from build123d import *

# Parameters (mm, degrees)
F0_W     = 20.5
F0_H     = 15.25
F0_W_2   = 18
F0_H_2   = 13
F0_R     = 3.125
F1_DEPTH = 2
F2_DEPTH = 5


# Not quite as in the source:
# - a fillet or chamfer that OpenCascade refuses, or shapes differently, is made with other operations: its cross-section is extruded or revolved along the edge and cut away or added


with BuildPart() as f1:
    # F0 (on Top) → F1 (new body)
    with BuildSketch(Plane.XY):
        Rectangle(F0_W, F0_H)
        Rectangle(F0_W_2, F0_H_2, mode=Mode.SUBTRACT)
        Rectangle(F0_W_2, F0_H_2)
        with Locations((-1.775, -3.075)):
            Circle(F0_R, mode=Mode.SUBTRACT)
        with Locations((5.475, -3.075)):
            Circle(F0_R, mode=Mode.SUBTRACT)
        with Locations((-5.475, 3.075)):
            Circle(F0_R, mode=Mode.SUBTRACT)
        with Locations((1.775, 3.075)):
            Circle(F0_R, mode=Mode.SUBTRACT)
    extrude(amount=F1_DEPTH)

    # F0 (on Top) → F2 (join)
    with BuildSketch(Plane.XY):
        Rectangle(F0_W_2, F0_H_2)
        with Locations((-1.775, -3.075)):
            Circle(F0_R, mode=Mode.SUBTRACT)
        with Locations((5.475, -3.075)):
            Circle(F0_R, mode=Mode.SUBTRACT)
        with Locations((-5.475, 3.075)):
            Circle(F0_R, mode=Mode.SUBTRACT)
        with Locations((1.775, 3.075)):
            Circle(F0_R, mode=Mode.SUBTRACT)
    extrude(amount=F2_DEPTH)

    # F3: fillet of radius 1 on 4 edges, made by hand

    # F3_s1 → F3_t2 (revolve, cut)
    with BuildSketch(Plane.XZ.offset(-3.075)):
        with BuildLine():
            ThreePointArc((-1.35, 5), (-2.0571067812, 4.7071067812), (-2.35, 4))
            Line((-2.35, 4), (-2.35, 5))
            Line((-2.35, 5), (-1.35, 5))
        make_face()
    revolve(axis=Axis((-5.475, 3.075, 5), (0, 0, 1)), mode=Mode.SUBTRACT)

    # F3_s3 → F3_t4 (revolve, cut)
    with BuildSketch(Plane.XZ.offset(-3.075)):
        with BuildLine():
            ThreePointArc((5.9, 5), (5.1928932188, 4.7071067812), (4.9, 4))
            Line((4.9, 4), (4.9, 5))
            Line((4.9, 5), (5.9, 5))
        make_face()
    revolve(axis=Axis((1.775, 3.075, 5), (0, 0, 1)), mode=Mode.SUBTRACT)

    # F3_s5 → F3_t6 (revolve, cut)
    with BuildSketch(Plane.XZ.offset(3.075)):
        with BuildLine():
            ThreePointArc((2.35, 5), (1.6428932188, 4.7071067812), (1.35, 4))
            Line((1.35, 4), (1.35, 5))
            Line((1.35, 5), (2.35, 5))
        make_face()
    revolve(axis=Axis((-1.775, -3.075, 5), (0, 0, 1)), mode=Mode.SUBTRACT)

    # F3_s7 → F3_t8 (revolve, cut)
    with BuildSketch(Plane.XZ.offset(3.075)):
        with BuildLine():
            ThreePointArc((9.6, 5), (8.8928932188, 4.7071067812), (8.6, 4))
            Line((8.6, 4), (8.6, 5))
            Line((8.6, 5), (9.6, 5))
        make_face()
    revolve(axis=Axis((5.475, -3.075, 5), (0, 0, 1)), mode=Mode.SUBTRACT)


solid = f1.part
Read the model definition and answer for the solid it produces. Units are mm, in the model's axes. A direction names the side the tool comes from. Round coordinates to 2 decimals unless told otherwise and drop trailing zeros. Write each loop counter-clockwise with the first axis right and the second up, starting at its lowest first coordinate (ties: lowest second). Pieces come first, ordered by that corner, then holes.
1. The part is cut by section B-B, the plane y = 3.5. State how many separate pieces and enclosed holes the cut face has, then the cut area to 3 significant figures.
2. Determine the mould class of faces 1 (the face through (4.662, 1.878, 1.972)), 2 (the face through (-9, 0, 3)), 3 (the face through (-2, 6, 5)) for opening direction X: pulls with the +X half, pulls with the -X half, needs draft (parallel to the pull), parting line crosses it, or undercut.
3. The part is cut by section A-A, the plane z = 3.6. Determine the outline of the cut face in (x, y) (3 decimals).
4. Which of the six approach directions +Z, -Z, +X, -X, +Y, -Y give full straight-line access (tool end or side, diameter ignored) to faces 4 (the face through (9, 0, 3)), 5 (the face through (0, 7, 2)), 6 (the face through (0, -6.5, 3))?
5. Given pin 1 Ø5.5 at (x, y) = (5.475, -3.075) entering from +Z; pin 2 Ø0.9 at (y, z) = (1.5, 3.5) entering from -X; pin 3 Ø2.5 at (x, z) = (3.5, 3.5) entering from +Y; pin 4 Ø1.5 at (x, z) = (3.5, 4) entering from -Y, each flat-ended and moving along its own axis, determine where each tip first touches the part or whether it passes through.
6. Straight lines are drawn through the part: L1, parallel to Y at x = 5.5, z = 1.7 (3 decimals); L2, parallel to X at y = -2, z = 1.6; L3, parallel to X at y = 4, z = 4.1. For each, find the intervals that lie inside material, in ascending order.
Values:
1. separate pieces: 3
1. enclosed holes: 0
1. area: 32.3 mm2
2. face 1: undercut
2. face 2: pulls with the -X half
2. face 3: needs draft
3. outline: (-9, -6.5) - (9, -6.5) - (9, 6.5) - (-9, 6.5) - close; hole circle Ø6.25 at (-5.475, 3.075); hole circle Ø6.25 at (-1.775, -3.075); hole circle Ø6.25 at (1.775, 3.075); hole circle Ø6.25 at (5.475, -3.075)
4. face 4: +Z, +X, +Y, -Y
4. face 5: +Z
4. face 6: +Z, +X, -X, -Y
5. pin 1: passes through
5. pin 2: stops at x = -9
5. pin 3: stops at y = 6.5
5. pin 4: stops at y = -6.5
6. L1: y = -7.625 to -6.2, 0.05 to 7.625
6. L2: x = -10.25 to -4.71, 1.16 to 2.54, 8.41 to 10.25
6. L3: x = -9 to -8.47, -2.48 to -1.22, 4.77 to 9
